Verification items for the finished model (mm, model axes). Face numbers are marked on the shaded views. A direction names the side the tool comes from. Coordinates: 2 decimals unless noted, no trailing zeros. Write each loop counter-clockwise with the first axis right and the second up, starting at its lowest first coordinate (ties: lowest second). Pieces come first, ordered by that corner, then holes. Notation, with made-up numbers: (58, -25.5) -> (63, -25.5) arc R24 cw to (63, 11.5) -> close; hole circle Ø3 at (22.5, 66.5). An arc over 180 degrees is marked (long way). Answer in a Markdown table with one row per item.
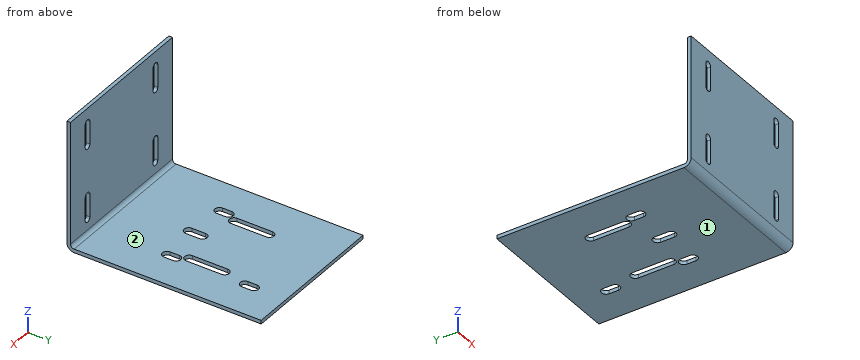
Autodesk Inventor part; units mm, degrees
ref_plane "YZ Plane" through (0, 0, 0) normal (1, 0, 0) x (0, 1, 0)
ref_plane "XZ Plane" through (0, 0, 0) normal (0, 1, 0) x (-1, 0, 0)
ref_plane "XY Plane" through (0, 0, 0) normal (0, 0, 1) x (1, 0, 0)
sketch "Sketch1" plane through (0, 0, 0) normal (0, 1, 0) x (-1, 0, 0)
  line L0 (33, -27.5) -> (-33, -27.5)
  line L1 (-33, -27.5) -> (-33, 27.5)
  line L2 (-33, 27.5) -> (33, 27.5)
  line L3 (33, 27.5) -> (33, -27.5)
  line L4 (33, -27.5) -> (-33, 27.5) construction
  line L5 (-33, -27.5) -> (33, 27.5) construction
  point P0 (0, 0)
  dimension "d0" = 66
  dimension "d1" = 55
extrude "Plate1" add sketch "Sketch1" along normal blind 1.5875
sketch "Sketch3" plane through (0, 1.5875, 0) normal (0, 1, 0) x (1, 0, 0)
  line L0 (0, 0) -> (-33, 0)
  line L1 (-33, 0) -> (-33, 27.5)
  line L2 (-33, 27.5) -> (0, 27.5)
  line L3 (0, 27.5) -> (0, 0)
  circle A0 centre (-22, 16) radius 1.5
  circle A1 centre (-22, -16) radius 1.5
  circle A2 centre (22, 16) radius 1.5
  circle A3 centre (22, -16) radius 1.5
  line L4 (-22, 11) -> (-22, 21) construction
  line L5 (-20.5, 11) -> (-20.5, 21)
  line L6 (-23.5, 21) -> (-23.5, 11)
  arc A4 (-23.5, 11) -> (-20.5, 11) centre (-22, 11) ccw
  arc A5 (-20.5, 21) -> (-23.5, 21) centre (-22, 21) ccw
  line L7 (20.5, 11) -> (20.5, 21)
  line L8 (23.5, 21) -> (23.5, 11)
  arc A6 (20.5, 11) -> (23.5, 11) centre (22, 11) ccw
  arc A7 (23.5, 21) -> (20.5, 21) centre (22, 21) ccw
  line L9 (-20.5, -11) -> (-20.5, -21)
  line L10 (-23.5, -21) -> (-23.5, -11)
  arc A8 (-20.5, -11) -> (-23.5, -11) centre (-22, -11) ccw
  arc A9 (-23.5, -21) -> (-20.5, -21) centre (-22, -21) ccw
  arc A10 (20.5, -21) -> (23.5, -21) centre (22, -21) ccw
  line L11 (23.5, -21) -> (23.5, -11)
  line L12 (20.5, -11) -> (20.5, -21)
  arc A11 (23.5, -11) -> (20.5, -11) centre (22, -11) ccw
  dimension "d22" = 3
  dimension "d23" = 32
  dimension "d24" = 22
  dimension "d48" = 5
  dimension "d49" = 3
extrude "Cut1" cut sketch "Sketch3" against normal blind 1.5875 contours A0 | L5 A4 L6 A0 | A0 L6 A5 L5 | A1 | L9 A9 L10 A1 | A1 L10 A8 L9 | A2 | L8 A6 L7 A2 | A2 L7 A7 L8 | A3 | L11 A10 L12 A3 | A3 L12 A11 L11
sketch "Sketch2" plane through (-33, 1.5875, -27.5) normal (0, 0, -1) x (-1, 0, 0)
  line L0 (-66, 0) -> (0, 0)
  line L1 (0, 0) -> (0, 83.4125)
  line L2 (0, 83.4125) -> (-66, 83.4125)
  line L3 (-66, 83.4125) -> (-66, 0)
edge flange "Flange1" height 85 angle 90 thickness 1.5875 bend radius 1.5875 thickness toward (0, 0, -1) relief tear relief width 1.5875 relief depth 0.7937 edges at (0, 1.5875, -27.5) wall of the first edge with corners at (33, 1.5875, -27.5) (-33, 1.5875, -27.5) (-33, 85, -27.5) (33, 85, -27.5)
bend "Bend1"
corner "Corner1"
sketch "Sketch4" plane through (33, 85, -29.0875) normal (0, 0, -1) x (-1, 0, 0)
  line L0 (0, -81.825) -> (66, -81.825)
  line L1 (66, 0) -> (66, -81.825)
  line L2 (0, 0) -> (66, 0)
  line L3 (33, -54) -> (33, -48) construction
  line L4 (35, -54) -> (35, -48)
  line L5 (31, -48) -> (31, -54)
  arc A0 (31, -54) -> (35, -54) centre (33, -54) ccw
  arc A1 (35, -48) -> (31, -48) centre (33, -48) ccw
  line L6 (33, -81.825) -> (33, 0)
  line L7 (47.5, -44) -> (47.5, -28.5) construction
  line L8 (49.5, -44) -> (49.5, -28.5)
  line L9 (45.5, -28.5) -> (45.5, -44)
  arc A2 (45.5, -44) -> (49.5, -44) centre (47.5, -44) ccw
  arc A3 (49.5, -28.5) -> (45.5, -28.5) centre (47.5, -28.5) ccw
  line L10 (18.5, -44) -> (18.5, -28.5) construction
  line L11 (16.5, -44) -> (16.5, -28.5)
  line L12 (20.5, -28.5) -> (20.5, -44)
  arc A4 (16.5, -44) -> (20.5, -44) centre (18.5, -44) ccw
  arc A5 (20.5, -28.5) -> (16.5, -28.5) centre (18.5, -28.5) ccw
  line L13 (66, -85) -> (0, -85)
  line L14 (16, -50) -> (50, -50)
  line L15 (50, -50) -> (50, -16)
  line L16 (50, -16) -> (16, -16)
  line L17 (16, -16) -> (16, -50)
  circle A6 centre (16, -16) radius 2
  circle A7 centre (16, -50) radius 2
  circle A8 centre (50, -50) radius 2
  line L18 (33, -16) -> (33, -50)
  line L19 (16, -18) -> (16, -14) construction
  line L20 (18, -18) -> (18, -14)
  line L21 (14, -14) -> (14, -18)
  arc A9 (14, -18) -> (18, -18) centre (16, -18) ccw
  arc A10 (18, -14) -> (14, -14) centre (16, -14) ccw
  line L22 (16, -52) -> (16, -48) construction
  line L23 (18, -52) -> (18, -48)
  line L24 (14, -48) -> (14, -52)
  arc A11 (14, -52) -> (18, -52) centre (16, -52) ccw
  arc A12 (18, -48) -> (14, -48) centre (16, -48) ccw
  line L25 (50, -52) -> (50, -48) construction
  line L26 (52, -52) -> (52, -48)
  line L27 (48, -48) -> (48, -52)
  arc A13 (48, -52) -> (52, -52) centre (50, -52) ccw
  arc A14 (52, -48) -> (48, -48) centre (50, -48) ccw
  point P0 (33, -85)
  point P1 (33, -51)
  point P2 (47.5, -36.25)
  point P3 (18.5, -36.25)
  dimension "d25" = 3
  dimension "d26" = 4
  dimension "d29" = 4
  dimension "d30" = 15.5
  dimension "d31" = 14.5
  dimension "d46" = 48.75
  dimension "d47" = 34
  dimension "d50" = 34
  dimension "d51" = 34
  dimension "d52" = 4
  dimension "d53" = 4
  dimension "d54" = 4
  dimension "d55" = 35
  dimension "d56" = 0
  dimension "d57" = 2
  dimension "d58" = 4
  dimension "d59" = 2
  dimension "d60" = 4
  dimension "d61" = 2
  dimension "d62" = 4
extrude "Cut2" cut sketch "Sketch4" against normal blind 1.5875 contours L6 L14 L4 A0 | A0 L5 L14 L6 | L14 L5 A1 L6 | L6 A1 L4 L14 | A7 L17 L14 | L14 L17 A7 | L23 A11 L24 A7 | A7 L17 A12 L23 | A8 L15 L14 | L27 A14 L15 A8 | L14 L15 A8 | A8 L26 A13 L27 | A6 L17 L16 | L16 L17 A6 | L20 A9 L17 A6 | A6 L21 A10 L20 | A7 L24 A12 L17 | L15 A14 L26 A8 | A6 L17 A9 L21 | A2 L9 A3 L8 | L11 A5 L12 A4
equation "\"d0\" = subframe_x"
equation "\"d1\" = subframe_y"
equation "\"d22\" = m3_diameter"
equation "\"d23\" = 0.4 * frame_y"
equation "\"d24\" = 0.333333 * subframe_x"
equation "\"d49\" = m3_diameter"
equation "\"d20\" = Thickness"
equation "\"d26\" = m4_diameter"
equation "\"d29\" = m4_diameter"
equation "\"d33\" = Thickness"
equation "\"Thickness\" = sm_thickness"
equation "\"d3\" = BendReliefWidth"
equation "\"d4\" = BendReliefDepth"
equation "\"d5\" = MinimumRemnant"
equation "\"d6\" = BendRadius"
equation "\"d7\" = galvo_frame_z"
equation "\"d9\" = BendRadius"
equation "\"d11\" = CornerReliefSize"
equation "\"d12\" = GapSize"
equation "\"d13\" = JacobiRadiusSize"
equation "\"BendRadius\" = Thickness"
equation "\"BendReliefWidth\" = Thickness"
equation "\"BendReliefDepth\" = 0.5 * Thickness"
equation "\"CornerReliefSize\" = 4 * Thickness"
equation "\"MinimumRemnant\" = 2 * Thickness"
equation "\"TransitionRadius\" = BendRadius"
equation "\"JacobiRadiusSize\" = BendRadius"
equation "\"GapSize\" = Thickness"
equation "\"sm_thickness\" = 1.5875"
equation "\"very_thick_acrylic\" = 9.45"
equation "\"thick_acrylic\" = 5.88"
equation "\"thin_acrylic\" = 3.15"
equation "\"clear_acrylic\" = 3.15"
equation "\"wood_thickness\" = 6.72"
equation "\"m3_diameter\" = 3"
equation "\"m3_head\" = 6"
equation "\"m4_diameter\" = 4"
equation "\"m5_diameter\" = 5"
equation "\"m5_head\" = 10.3"
equation "\"brass_insert_drill\" = 4"
equation "\"m5_brass_insert_drill\" = 6.7"
equation "\"m3_press_nut_drill\" = 4.5"
equation "\"m5_press_nut_drill\" = 6.5"
equation "\"laser_body_diameter\" = 12"
equation "\"carrier_y\" = 251"
equation "\"carrier_z\" = 12"
equation "\"visor_x\" = 253.925"
equation "\"visor_y\" = 85.6"
equation "\"window_z\" = 332.225"
equation "\"window_y\" = 93.75"
equation "\"window_overlap\" = 48"
equation "\"acrylic_into_frame\" = 5"
equation "\"door_x\" = 251"
equation "\"door_z\" = 332.225"
equation "\"door_overlap\" = 48"
equation "\"reservoir_x\" = 201"
equation "\"reservoir_y\" = 201"
equation "\"linear_bearing_spacing\" = 271"
equation "\"tray_border\" = 25"
equation "\"tray_x\" = 251"
equation "\"tray_y\" = 251"
equation "\"bed_z\" = 25"
equation "\"crane_z2\" = 12"
equation "\"switch_spacing\" = 19"
equation "\"frame_top_z\" = 385"
equation "\"frame_bottom_z\" = 275"
equation "\"frame_total_z\" = 661.5875"
equation "\"frame_face_y\" = 45"
equation "\"frame_border\" = 48.0375"
equation "\"frame_foot_z\" = 12"
equation "\"frame_screw_from_center\" = 25"
equation "\"laser_y_offset\" = 19.4"
equation "\"laser_diameter\" = 12"
equation "\"laser_z_offset\" = 55"
equation "\"laser_y\" = 15"
equation "\"laser_z\" = 75"
equation "\"laser_gap\" = 1"
equation "\"subframe_x\" = 66"
equation "\"subframe_y\" = 55"
equation "\"galvo_frame_x\" = 66"
equation "\"galvo_frame_z\" = 85"
equation "\"galvo_frame_y_offset\" = 27.5"
equation "\"drawer_x\" = 257.3"
equation "\"drawer_y\" = 90.3375"
equation "\"drawer_z\" = 278.175"
equation "\"drawer_support_from_top\" = 48"
equation "\"drawer_screw_from_center\" = 55"
equation "\"nema17_x\" = 43"
equation "\"d2\" = BendRadius"
equation "\"d44\" = galvo_frame_x"
equation "\"al_thickness\" = 1.5875"
equation "\"rivet_diameter\" = 3.3"
equation "\"bend_factor\" = 2.26205"
equation "\"sm_bend\" = 3.591"
equation "\"al_bend\" = 3.591"
equation "\"frame_x\" = 353.375"
equation "\"carrier_z2\" = 25"
equation "\"carrier_y2\" = 76.825"
properties part number "subframe"
1. Access from +Z, -Z, +X, -X, +Y, -Y to the whole of each face (thin tool, end or side, straight path). Record for the marked faces 1 and 2.
Findings below:
| item | result |
|---|---|
| face 1 | -Z, +X, -X, +Y, -Y |
| face 2 | +Z, +X, -X, +Y |
2. Sectioned sample at C-C, the plane y = 45.5. Record the cut outline in (x, z).
Findings below:
| item | result |
|---|---|
| outline | (-33, -29.09) -> (-16.5, -29.09) -> (-16.5, -27.5) -> (-33, -27.5) -> close; (-12.5, -29.09) -> (12.5, -29.09) -> (12.5, -27.5) -> (-12.5, -27.5) -> close; (16.5, -29.09) -> (33, -29.09) -> (33, -27.5) -> (16.5, -27.5) -> close |
3. Sectioned sample at A-A, the plane z = -19.5. Record the cut outline in (x, y), and give its area (4 significant figures).
Findings below:
| item | result |
|---|---|
| outline | (-33, 0) -> (-23.5, 0) -> (-23.5, 1.59) -> (-33, 1.59) -> close; (-20.5, 0) -> (20.5, 0) -> (20.5, 1.59) -> (-20.5, 1.59) -> close; (23.5, 0) -> (33, 0) -> (33, 1.59) -> (23.5, 1.59) -> close |
| area | 95.25 mm² |
4. Go/stop test with flat-tipped pins: pin 1 (8 mm diameter, centred on x = 20, z = 7.5, fed in from +Y); pin 2 (2 mm diameter, centred on x = -25, z = -6.5, fed in from -Y); pin 3 (20 mm diameter, centred on x = 7, y = 45, fed in from +Z). Record where each tip stops, or that it passes through.
Findings below:
| item | result |
|---|---|
| pin 1 | stops at y = 1.59 |
| pin 2 | stops at y = 0 |
| pin 3 | stops at z = -27.5 |
5. Material ranges on probe 1 along Y at (x, z) = (-20, -10.5); probe 2 along Z at (x, y) = (-22.5, 65.5), recorded low to high. Write a range as from..to.
Findings below:
| item | result |
|---|---|
| probe 1 | y = 0..1.59 |
| probe 2 | z = -29.09..-27.5 |
6. Sectioned sample at B-B, the plane x = 22. Count the separate pieces of the cut face and the enclosed holes in it, and give its area (3 significant figures).
Findings below:
| item | result |
|---|---|
| separate pieces | 3 |
| enclosed holes | 0 |
| area | 179 mm² |
